Input: dimensioned drawing with shaded views. Units: mm. Origin: part minimum x, y, z. A direction names the side the tool comes from. Round coordinates to 2 decimals unless told otherwise and drop trailing zeros. Write each loop counter-clockwise with the first axis right and the second up, starting at its lowest first coordinate (ties: lowest second). Pieces come first, ordered by that corner, then holes. Notation, with made-up numbers: M 47,86.25 L 103,86.25 A19 ccw 103,104.25 Z; hole C -13.75,23 d4. An arc over 180 degrees is marked long. Use one line per item in the form item = value. Start each with the question number.
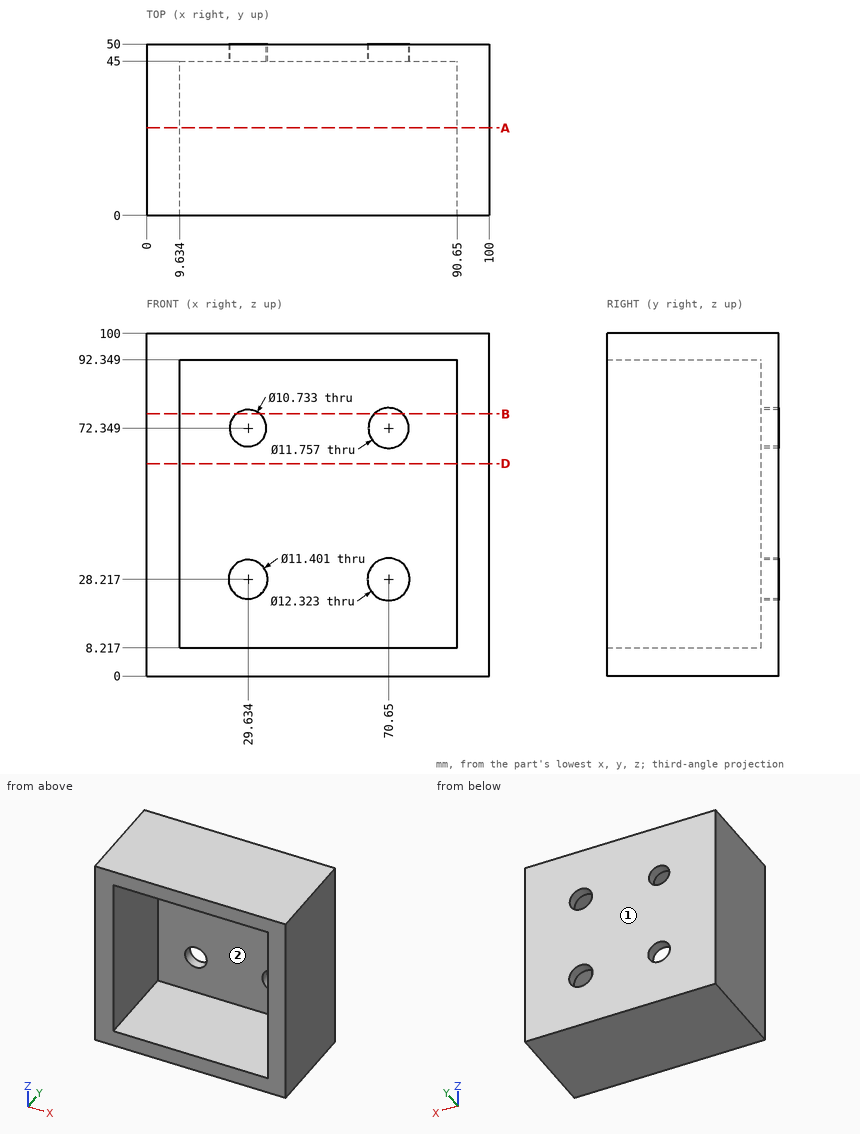
1. Section query A-A (y = 25.5). Return loops of the section in (x, z).
2. Ray query, probe 1 along X at (y, z) = (35.5, 37); probe 2 along Z at (x, y) = (89.5, 44.5); probe 3 along Y at (x, z) = (46.5, 42.5). Return the intervals inside material, ascending.
3. Section query D-D (z = 62). Return loops of the section in (x, y).
4. Set-up query: the marked faces 1 and 2. Return all of +Z, -Z, +X, -X, +Y, -Y with unobstructed straight access to the full face (end or side cutting, diameter ignored); none if empty.
5. Section query B-B (z = 76.5). Give the number of separate pieces and of enclosed holes in the cut face, then the cut area to 3 significant figures.
6. Contact query for a flat-ended pin moving along its axis: pin 1 (4 mm diameter, centred on x = 14.5, z = 27, fed in from -Y). Output: stop coordinate, or through.
Checks:
q1.outline = M 0,0 L 100,0 L 100,100 L 0,100 Z; hole M 9.63,8.22 L 90.65,8.22 L 90.65,92.35 L 9.63,92.35 Z
q2.probe_1 = 0 to 9.63, 90.65 to 100
q2.probe_2 = 0 to 8.22, 92.35 to 100
q2.probe_3 = 45 to 50
q3.outline = M 0,0 L 9.63,0 L 9.63,45 L 90.65,45 L 90.65,0 L 100,0 L 100,50 L 0,50 Z
q4.face_1 = +Z, -Z, +X, -X, +Y
q4.face_2 = -Y
q5.separate_pieces = 3
q5.enclosed_holes = 0
q5.area = 1,280 mm^2
q6.pin_1 = 45
